```python
from build123d import *

# Parameters (mm, degrees)
ESBO_O1_R                = 4
ESBO_O1_W                = 11
ESBO_O1_H                = 4
RESSALTO_EXTRUS_O1_DEPTH = 10


with BuildPart() as part:
    # Esboço1 → Ressalto-extrusão1 (new body)
    with BuildSketch(Plane.XY):
        with BuildLine():
            Line((4, 6.34428877), (4, 63.65571123))
            ThreePointArc((4, 63.65571123), (0, 77.5), (-4, 63.65571123))
            Line((-4, 63.65571123), (-4, 54))
            Line((-4, 54), (-19, 54))
            Line((-19, 54), (-19, 42))
            Line((-19, 42), (-4, 42))
            Line((-4, 42), (-4, 6.34428877))
            ThreePointArc((-4, 6.34428877), (0, -7.5), (4, 6.34428877))
        make_face()
        Circle(ESBO_O1_R, mode=Mode.SUBTRACT)
        with Locations((-9.5, 48)):
            Rectangle(ESBO_O1_W, ESBO_O1_H, mode=Mode.SUBTRACT)
        with Locations((0, 70)):
            Circle(ESBO_O1_R, mode=Mode.SUBTRACT)
    extrude(amount=RESSALTO_EXTRUS_O1_DEPTH)


solid = part.part
```
Verification items for the finished model (mm, model axes). A direction names the side the tool comes from. Coordinates: 2 decimals unless noted, no trailing zeros. Write each loop counter-clockwise with the first axis right and the second up, starting at its lowest first coordinate (ties: lowest second). Pieces come first, ordered by that corner, then holes. Notation, with made-up numbers: M 69,-1.5 L 104,-1.5 A17 ccw 104,25.5 Z; hole C 26.25,67 d10. An arc over 180 degrees is marked long. Answer as a JSON object with one key per item and string values. Group by question number.
(1) Cross-section at C-C, the plane z = 7.25. Record the cut outline in (x, y).
(2) Material ranges on line 1 (Y direction, x = -14.25, z = 8.75); line 2 (Y direction, x = 0.25, z = 9.5); line 3 (Y direction, x = -4.5, z = 4), recorded low to high.
(3) Cross-section at D-D, the plane x = 0. Record the cut outline in (y, z), and give its area (3 significant figures).
(4) Cross-section at B-B, the plane x = -11. Record the cut outline in (y, z).
(5) Tool access check on faces 1 (the face through (4, 35, 5)), 2 (the face through (-10, 46, 5)), 3 (the face through (-12, 42, 5)). Record the directions out of +Z, -Z, +X, -X, +Y, -Y that give a thin tool (end or side, any length) a straight path to the whole face; none if there is none.
(6) Gauge pin test, flat ends, axial feed: pin 1 (6 mm diameter, centred on y = 32.5, z = 3, fed in from +X); pin 2 (3 mm diameter, centred on x = -11, z = 4.5, fed in from -Y); pin 3 (1.5 mm diameter, centred on y = 56.5, z = 7, fed in from -X). Record the tip position at first contact, or that the pin passes through.
(7) Cross-section at A-A, the plane y = 0. Record the cut outline in (x, z).
Reply:
{
 "1": {"outline": "M -19,42 L -4,42 L -4,6.34 A7.5 ccw long 4,6.34 L 4,63.66 A7.5 ccw long -4,63.66 L -4,54 L -19,54 Z; hole M -15,46 L -4,46 L -4,50 L -15,50 Z; hole C 0,0 d8; hole C 0,70 d8"},
 "2": {"line 1": "42 to 46, 50 to 54", "line 2": "-7.5 to -3.99, 3.99 to 66.01, 73.99 to 77.5", "line 3": "-6 to 6, 42 to 46, 50 to 54, 64 to 76"},
 "3": {"outline": "M -7.5,0 L -4,0 L -4,10 L -7.5,10 Z; M 4,0 L 66,0 L 66,10 L 4,10 Z; M 74,0 L 77.5,0 L 77.5,10 L 74,10 Z", "area": "690 mm²"},
 "4": {"outline": "M 42,0 L 46,0 L 46,10 L 42,10 Z; M 50,0 L 54,0 L 54,10 L 50,10 Z"},
 "5": {"face 1": "+Z, -Z, +X", "face 2": "+Z, -Z", "face 3": "+Z, -Z, -X"},
 "6": {"pin 1": "x = 4", "pin 2": "y = 42", "pin 3": "x = -4"},
 "7": {"outline": "M -7.5,0 L -4,0 L -4,10 L -7.5,10 Z; M 4,0 L 7.5,0 L 7.5,10 L 4,10 Z"}
}
